from build123d import *

# Parameters (mm, degrees)
EXTRUDE_1_DEPTH     = 13
SKETCH_3_W          = 60
SKETCH_3_H          = 30
EXTRUDE_2_DEPTH     = 50
CHAMFER_1_SIZE      = 5
SKETCH_4_R          = 6.5
SKETCH_4_R_2        = 5
CUT_EXTRUDE_1_DEPTH = 50
SKETCH_5_R          = 10
CUT_EXTRUDE_2_DEPTH = 50


with BuildPart() as part:
    # Эскиз1 → Бобышка-Вытянуть1 (new body)
    with BuildSketch(Plane(origin=(0, 0, 0), x_dir=(1, 0, 0), z_dir=(0, 1, 0))):
        Polygon((0, 70), (10, 80), (100, 80), (110, 70), (110, 10), (100, 0), (10, 0), (0, 10), align=None)
    extrude(amount=EXTRUDE_1_DEPTH)

    # Эскиз3 → Бобышка-Вытянуть2 (add)
    with BuildSketch(Plane(origin=(0, 13, 0), x_dir=(1, 0, 0), z_dir=(0, 1, 0))):
        with Locations((55, 40)):
            Rectangle(SKETCH_3_W, SKETCH_3_H)
    extrude(amount=EXTRUDE_2_DEPTH)

    # Фаска1
    chamfer_1_edges = [part.edges().sort_by_distance(p)[0] for p in [
        (25, 63, -40),
        (85, 63, -40),
    ]]
    chamfer(chamfer_1_edges, length=CHAMFER_1_SIZE)

    # Эскиз4 → Вырез-Вытянуть1 (cut)
    with BuildSketch(Plane(origin=(0, 13, 0), x_dir=(1, 0, 0), z_dir=(0, 1, 0))):
        with Locations((15, 65)):
            Circle(SKETCH_4_R)
        with Locations((95, 15)):
            Circle(SKETCH_4_R)
        with Locations((95, 65)):
            Circle(SKETCH_4_R_2)
        with Locations((15, 15)):
            Circle(SKETCH_4_R_2)
    extrude(amount=-CUT_EXTRUDE_1_DEPTH, mode=Mode.SUBTRACT)

    # Эскиз5 → Вырез-Вытянуть2 (cut)
    with BuildSketch(Plane.XY.offset(-25)):
        with Locations((55, 48)):
            Circle(SKETCH_5_R)
    extrude(amount=-CUT_EXTRUDE_2_DEPTH, mode=Mode.SUBTRACT)


solid = part.part
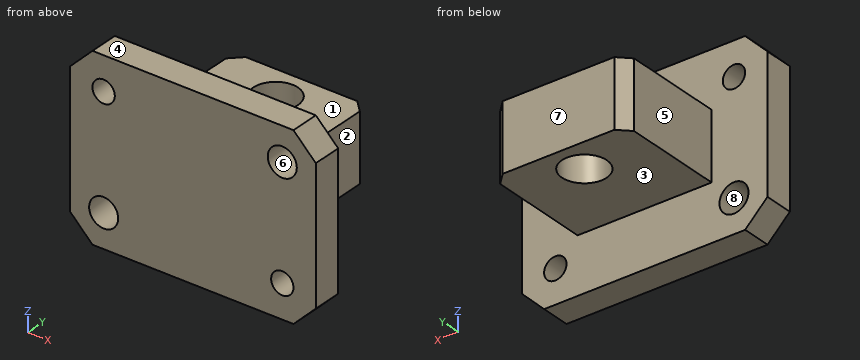
Input: part model. Units: mm. Frame: model coordinates. Face numbers are marked on the shaded views. A direction names the side the tool comes from. Round coordinates to 2 decimals unless told otherwise and drop trailing zeros. Order: outer loops, then holes, each group sorted by start corner. A loop starts at its lowest first (then second) coordinate and runs counter-clockwise, first axis right, second up. Notation, with made-up numbers: (76.25, 69.25) - (82.25, 69.25) arc R7 ccw to (82.25, 77.25) - close; hole circle Ø2 at (-23, 71). An arc over 180 degrees is marked (long way). Answer as a JSON object with one key per item and string values. Group by question number.
(1) Draft query along X for the marked faces 5, 6, 7 and 8. Return one class per face: released by +X, released by -X, zero draft, split by the parting line, or undercut.
(2) Pin query (flat end, axial travel): P1, Ø5, axis at x = 20.5, z = -40.5, coming from the +Y side; P2, Ø1.5, axis at x = 70, y = 48, coming from the +Z side; P3, Ø24, axis at y = 45, z = -33, coming from the -X side. Return the tip coordinate at first contact, or that it passes through.
(3) Reachability of the marked faces 1, 2, 3 and 4 from +Z, -Z, +X, -X, +Y, -Y: full face, straight path, thin tool, end or side. Return the list, or none.
(4) Cut plane B-B (z = -65). Return loops of the section in (x, y), then the cut area to 3 significant figures.
(5) Cut plane A-A (x = 95). Return loops of the section in (y, z).
(6) Cut plane C-C (y = 10). Return loops of the section in (x, z), then the cut area to 3 significant figures.
(7) Cut plane D-D (x = 62). Return loops of the section in (y, z).
(8) Material intervals for probe 1 along Z at (x, y) = (15, 8); probe 2 along Z at (x, y) = (95, 10.5); probe 3 along X at (y, z) = (9.25, -65), sorted ascending. Write a range as from..to.
Here are the results:
{
 "1": {"face 5": "released by -X", "face 6": "undercut", "face 7": "zero draft", "face 8": "undercut"},
 "2": {"P1": "stops at y = 13", "P2": "stops at z = -25", "P3": "stops at x = 25"},
 "3": {"face 1": "+Z, +X, -X, +Y", "face 2": "+Z, -Z, +X, +Y", "face 3": "-Z, +X, -X, +Y", "face 4": "+Z, +X, -X, +Y, -Y"},
 "4": {"outline": "(0, 0) - (8.5, 0) - (8.5, 13) - (0, 13) - close; (21.5, 0) - (90, 0) - (90, 13) - (21.5, 13) - close; (100, 0) - (110, 0) - (110, 13) - (100, 13) - close", "area": "1,130 mm^2"},
 "5": {"outline": "(0, -80) - (13, -80) - (13, -70) - (0, -70) - close; (0, -60) - (13, -60) - (13, -21.5) - (0, -21.5) - close; (0, -8.5) - (13, -8.5) - (13, 0) - (0, 0) - close"},
 "6": {"outline": "(0, -70) - (10, -80) - (100, -80) - (110, -70) - (110, -10) - (100, 0) - (10, 0) - (0, -10) - close; hole circle Ø13 at (15, -65); hole circle Ø10 at (15, -15); hole circle Ø13 at (95, -15); hole circle Ø10 at (95, -65)", "area": "8,180 mm^2"},
 "7": {"outline": "(0, -80) - (13, -80) - (13, -55) - (40.86, -55) - (40.86, -25) - (13, -25) - (13, 0) - (0, 0) - close; (55.14, -55) - (63, -55) - (63, -25) - (55.14, -25) - close"},
 "8": {"probe 1": "z = -80..-71.5, -58.5..-20, -10..0", "probe 2": "z = -80..-70, -60..-21.5, -8.5..0", "probe 3": "x = 0..8.5, 21.5..90, 100..110"}
}
